```python
from build123d import *

# Parameters (mm, degrees)
F0_R     = 6.1341
F1_DEPTH = 11.2522
F3_DEPTH = 8.636
F5_DEPTH = 25.4


with BuildPart() as f1:
    # F0 (on Top) → F1 (new body)
    with BuildSketch(Plane.XY):
        Circle(F0_R)
    extrude(amount=F1_DEPTH)

    # F2 (on face) → F3 (cut)
    with BuildSketch(Plane.XY.offset(11.2522)):
        Polygon((4.0894, -2.361016), (4.0894, 2.361016), (0, 4.722032), (-4.0894, 2.361016), (-4.0894, -2.361016), (0, -4.722032), align=None)
    extrude(amount=-F3_DEPTH, mode=Mode.SUBTRACT)

    # F4 (on face) → F5 (join)
    with BuildSketch(Plane(origin=(0, 0, 0), x_dir=(1, 0, 0), z_dir=(0, 0, -1))):
        Polygon((-1.81109, -3.1369), (1.81109, -3.1369), (3.62218, 0), (1.81109, 3.1369), (-1.81109, 3.1369), (-3.62218, 0), align=None)
    extrude(amount=F5_DEPTH)

    # F6 (on Front) → F7 (revolve)
    with BuildSketch(Plane.XZ):
        with BuildLine():
            Line((0, 0), (-3.62218, 0))
            Line((-3.62218, 0), (-3.62218, -8.7122))
            ThreePointArc((-3.62218, -8.7122), (-2.561268, -11.273468), (0, -12.33438))
            Line((0, -12.33438), (0, 0))
        make_face()
    revolve(axis=Axis((0, 0, -6.16719), (0, 0, -1)))


solid = f1.part
```
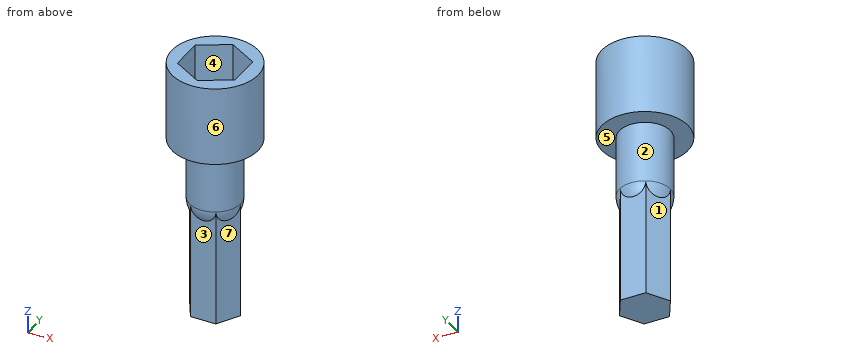
The listing builds one solid part. Answer for the finished solid, in the listing's coordinates (mm). Face numbers are marked on the shaded views. A direction names the side the tool comes from. Coordinates: 2 decimals unless noted, no trailing zeros. Write each loop counter-clockwise with the first axis right and the second up, starting at its lowest first coordinate (ties: lowest second). Pieces come first, ordered by that corner, then holes. Notation, with made-up numbers: (2, -7.75) - (55, -7.75) arc R20 cw to (55, 21.25) - close; hole circle Ø4 at (50, -17.75). An arc over 180 degrees is marked (long way). One line per item, written item: value.
1) Consider line 1 along Z through (x, y) = (-0.75, -4.75); line 2 along X through (y, z) = (3, 6); line 3 along Z through (x, y) = (1, 2). Determine where each line is inside the solid, lowest interval first. Write a range as from..to.
Geometry check:
line 1: z = 0..11.25
line 2: x = -5.35..-2.98, 2.98..5.35
line 3: z = -25.4..2.62
2) Find section B-B (z = -8). Give the vertices of the cut face in (x, y).
Geometry check:
outline: circle Ø7.24 at (0, 0)
3) For a pull along Y with two mould halves and no side action, classify the marked faces 1, 2, 3 and 4 as pulls with the +Y half, pulls with the -Y half, needs draft (parallel to the pull), parting line crosses it, or undercut.
Geometry check:
face 1: pulls with the +Y half
face 2: parting line crosses it
face 3: pulls with the -Y half
face 4: undercut
4) Each of these flat-tipped pins is pushed along its axis until it touches: pin 1 Ø1.5 at (x, z) = (4, -5) entering from -Y; pin 2 Ø1 at (x, y) = (3, 1.5) entering from -Z; pin 3 Ø3 at (x, z) = (0.5, -17.5) entering from -Y; pin 4 Ø3 at (x, z) = (-4, -2) entering from -Y. Where does it stop, or does it pass through?
Geometry check:
pin 1: stops at y = -1.6
pin 2: stops at z = -25.4
pin 3: stops at y = -3.14
pin 4: stops at y = -2.62
5) Find section A-A (z = -12.5). Give the vertices of the cut face in (x, y), and give its area (3 significant figures).
Geometry check:
outline: (-3.62, 0) - (-1.81, -3.14) - (1.81, -3.14) - (3.62, 0) - (1.81, 3.14) - (-1.81, 3.14) - close
area: 34.1 mm2
6) A tool of negligible diameter and unlimited length cuts with its end or side. For the marked faces 5, 6 and 7, from which of +Z, -Z, +X, -X, +Y, -Y can it reach the whole face along a straight path? Write none if from no direction.
Geometry check:
face 5: -Z
face 6: +Z, -Z
face 7: -Z, +X, -Y
